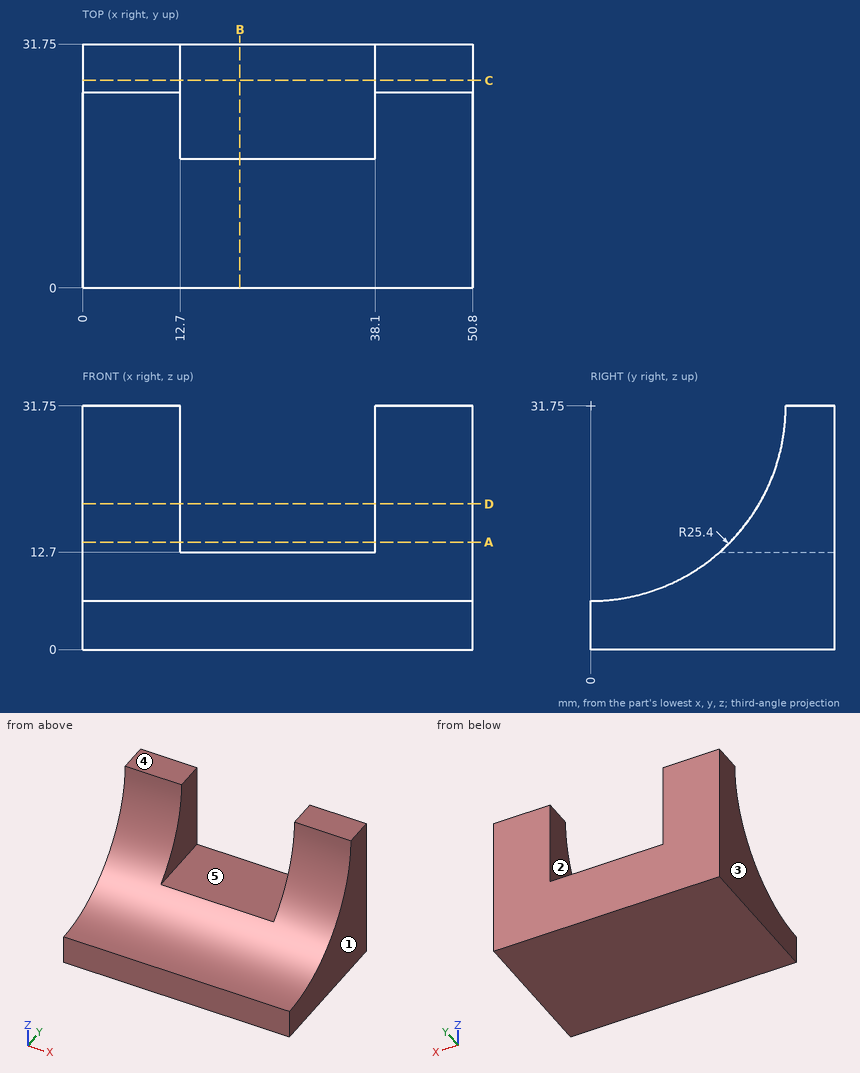
Geometry: see drawing. Coordinates: mm, zero at the bounding-box minimum. A direction names the side the tool comes from. Coordinates: 2 decimals unless noted, no trailing zeros. Write each loop counter-clockwise with the first axis right and the second up, starting at its lowest first coordinate (ties: lowest second). Pieces come first, ordered by that corner, then holes.
1) Set-up query: the marked faces 1 and 2. Return all of +Z, -Z, +X, -X, +Y, -Y with unobstructed straight access to the full face (end or side cutting, diameter ignored); none if empty.
2) Section A-A on z = 14. Output: boundary loops of the cut face in (x, y).
3) Mould query, pull axis X, two halves, no side actions, for the marked faces 3, 4 and 5. Classes: pulls with the +X half, pulls with the -X half, needs draft (parallel to the pull), parting line crosses it, or undercut.
4) Section B-B on x = 20.5. Output: boundary loops of the cut face in (y, z), and give its area (3 significant figures).
5) Section C-C on y = 27. Output: boundary loops of the cut face in (x, z), and give its area (3 significant figures).
6) Material intervals for line 1 along X through (y, z) = (22.5, 13); line 2 along Z through (x, y) = (31.5, 18); line 3 along Y through (x, z) = (14.5, 12.5), sorted ascending.
7) Pin query (flat end, axial travel): pin 1 Ø6 at (x, z) = (22.5, 14) entering from -Y; pin 2 Ø16.5 at (x, y) = (22.5, 23.5) entering from +Z. Return the tip coordinate at first contact, or that it passes through.
8) Section D-D on z = 19. Output: boundary loops of the cut face in (x, y), and give its area (3 significant figures).
Check result:
1. face 1: +Z, -Z, +X, +Y, -Y
1. face 2: +Z, +Y, -Y
2. outline: (0, 18.17) - (12.7, 18.17) - (12.7, 31.75) - (0, 31.75) - close; (38.1, 18.17) - (50.8, 18.17) - (50.8, 31.75) - (38.1, 31.75) - close
3. face 3: pulls with the -X half
3. face 4: needs draft
3. face 5: undercut
4. outline: (0, 0) - (31.75, 0) - (31.75, 12.7) - (16.8, 12.7) arc R25.4 cw to (0, 6.35) - close
4. area: 330 mm2
5. outline: (0, 0) - (50.8, 0) - (50.8, 31.75) - (38.1, 31.75) - (38.1, 12.7) - (12.7, 12.7) - (12.7, 31.75) - (0, 31.75) - close
5. area: 1,130 mm2
6. line 1: x = 0 to 12.7, 38.1 to 50.8
6. line 2: z = 0 to 12.7
6. line 3: y = 16.57 to 31.75
7. pin 1: stops at y = 14.65
7. pin 2: stops at z = 12.7
8. outline: (0, 21.97) - (12.7, 21.97) - (12.7, 31.75) - (0, 31.75) - close; (38.1, 21.97) - (50.8, 21.97) - (50.8, 31.75) - (38.1, 31.75) - close
8. area: 248 mm2
